Read the model definition and answer for the solid it produces. Units are mm, in the model's axes. Face numbers are marked on the shaded views. Round coordinates to 2 decimals unless told otherwise and drop trailing zeros. Loops run counter-clockwise (first coordinate to the right, second up) from the corner with the lowest first, then second, coordinate; pieces in that order, holes last. Notation, with made-up numbers: M 88,49 L 114,49 A20 cw 114,54 Z; hole C 27.5,65.25 d2. An arc over 180 degrees is marked long. Write each question's results on one line, items separated by ' | '.
from build123d import *

# Parameters (mm, degrees)
F0_R     = 40.5
F1_DEPTH = 40
F2_R     = 39.5
F3_DEPTH = 42
F4_R     = 5.70155
F5_DEPTH = 2


with BuildPart() as f1:
    # F0 (on Top) → F1 (new body)
    with BuildSketch(Plane.XY):
        Circle(F0_R)
    extrude(amount=F1_DEPTH)

    # F2 (on face) → F3 (cut)
    with BuildSketch(Plane.XY.offset(40)):
        Circle(F2_R)
    extrude(amount=-F3_DEPTH, mode=Mode.SUBTRACT)

    # F4 (on Top) → F5 (join)
    with BuildSketch(Plane.XY):
        with Locations((-40.165663, 0)):
            Circle(F4_R)
        with Locations((40.165663, 0)):
            Circle(F4_R)
    extrude(amount=F5_DEPTH)


solid = f1.part
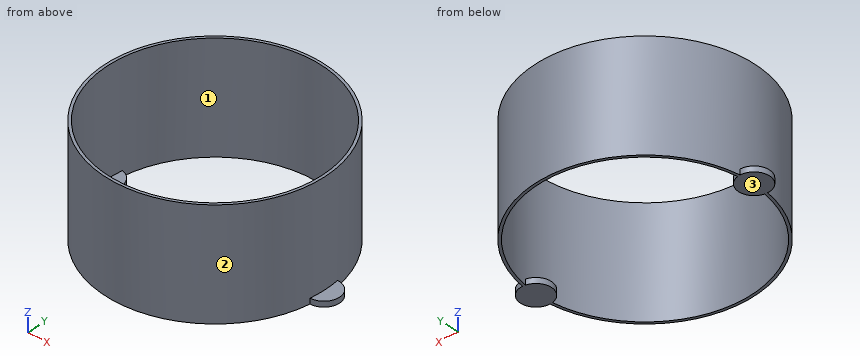
Item 1: The part is cut by section B-B (y = 0). Determine the outline of the cut face in (x, z), plus the area to 3 significant figures.
Outcome:
outline: M -45.87,0 L -34.46,0 L -34.46,2 L -39.5,2 L -39.5,40 L -40.5,40 L -40.5,2 L -45.87,2 Z; M 34.46,0 L 45.87,0 L 45.87,2 L 40.5,2 L 40.5,40 L 39.5,40 L 39.5,2 L 34.46,2 Z | area: 122 mm2
Item 2: The part is cut by section A-A (x = 0). Determine the outline of the cut face in (y, z).
Outcome:
outline: M -40.5,0 L -39.5,0 L -39.5,40 L -40.5,40 Z; M 39.5,0 L 40.5,0 L 40.5,40 L 39.5,40 Z
Item 3: Straight lines are drawn through the part: line 1 (Y direction, x = 0, z = 26.5); line 2 (X direction, y = -16, z = 26.5); line 3 (X direction, y = -29, z = 18). For each, find the intervals that lie inside material, in ascending order.
Outcome:
line 1: y = -40.5 to -39.5, 39.5 to 40.5 | line 2: x = -37.21 to -36.11, 36.11 to 37.21 | line 3: x = -28.27 to -26.82, 26.82 to 28.27
Item 4: The mould has two halves that part along Y. Classify the marked faces 1, 2 and 3: pulls with the +Y half, pulls with the -Y half, needs draft (parallel to the pull), parting line crosses it, or undercut.
Outcome:
face 1: undercut | face 2: parting line crosses it | face 3: needs draft
Item 5: The part is cut by section D-D (y = 11). Determine the outline of the cut face in (x, z), plus the area to 3 significant figures.
Outcome:
outline: M -38.98,0 L -37.94,0 L -37.94,40 L -38.98,40 Z; M 37.94,0 L 38.98,0 L 38.98,40 L 37.94,40 Z | area: 83.2 mm2
Item 6: The part is cut by section C-C (z = 18). Determine the outline of the cut face in (x, y).
Outcome:
outline: C 0,0 d81; hole C 0,0 d79
Item 7: Flat-ended cylindrical pins translate along their axes: pin 1 (6 mm diameter, centred on y = -2.5, z = 14, fed in from +X); pin 2 (3 mm diameter, centred on x = 33.5, z = 32, fed in from -Y); pin 3 (6 mm diameter, centred on x = 33.5, y = -30, fed in from -Z); pin 4 (3 mm diameter, centred on x = -44.5, y = -1, fed in from +Z). Find the tip coordinate at first contact, or state that the pin passes through.
Outcome:
pin 1: stops at x = 40.5 | pin 2: stops at y = -24.82 | pin 3: passes through | pin 4: stops at z = 2
